Geometry: see drawing. Coordinates: mm, zero at the bounding-box minimum. A direction names the side the tool comes from. Coordinates: 2 decimals unless noted, no trailing zeros. Write each loop counter-clockwise with the first axis right and the second up, starting at its lowest first coordinate (ties: lowest second). Pieces come first, ordered by that corner, then holes.
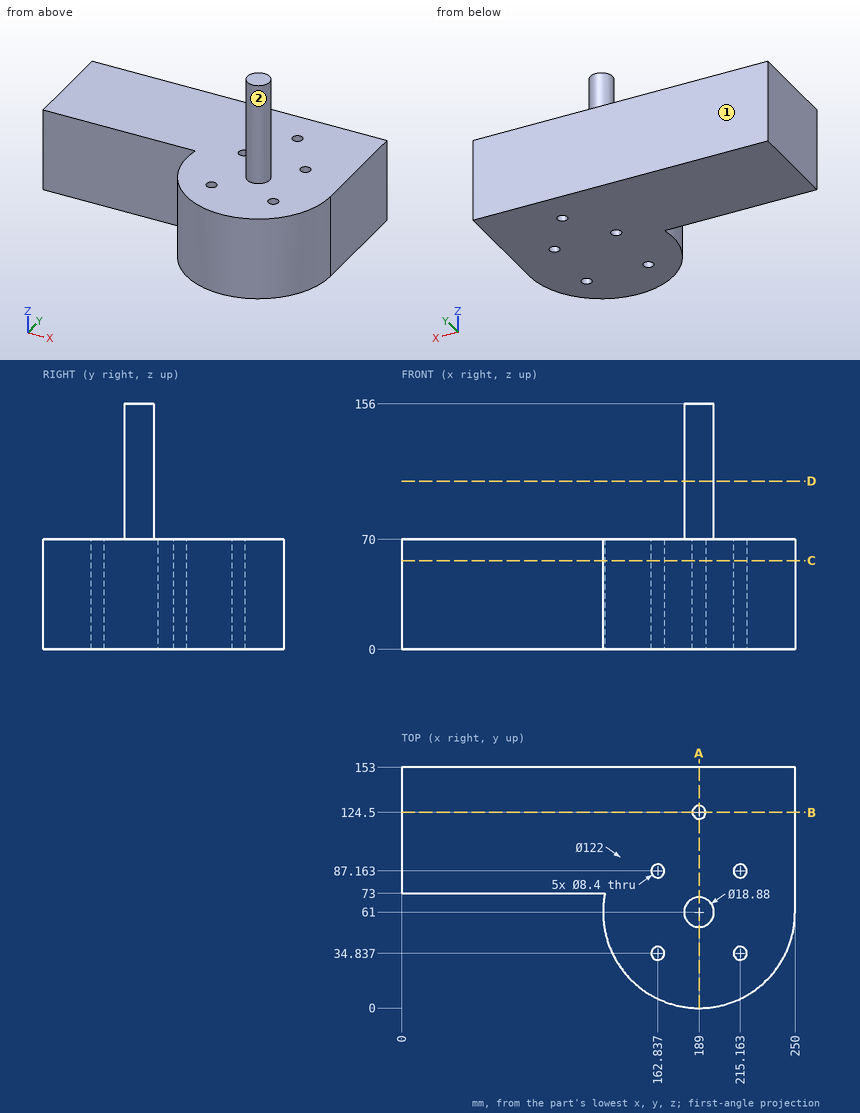
Item 1: Section A-A, the plane x = 189. Output: boundary loops of the cut face in (y, z).
Derived:
outline: (0, 0) - (120.3, 0) - (120.3, 70) - (70.44, 70) - (70.44, 156) - (51.56, 156) - (51.56, 70) - (0, 70) - close; (128.7, 0) - (153, 0) - (153, 70) - (128.7, 70) - close
Item 2: Set-up query: the marked faces 1 and 2. Return all of +Z, -Z, +X, -X, +Y, -Y with unobstructed straight access to the full face (end or side cutting, diameter ignored); none if empty.
Derived:
face 1: +Z, -Z, +X, -X, +Y
face 2: +Z
Item 3: Section D-D, the plane z = 107. Output: boundary loops of the cut face in (x, y), plus the area to 3 significant figures.
Derived:
outline: circle Ø18.88 at (189, 61)
area: 280 mm2
Item 4: Pin query (flat end, axial travel): pin 1 (13.5 mm diameter, centred on x = 215.16, y = 87.16, fed in from -Z); pin 2 (6 mm diameter, centred on x = 108, z = 36, fed in from -Y); pin 3 (1.5 mm diameter, centred on y = 58, z = 65.5, fed in from +X); pin 4 (6 mm diameter, centred on x = 33.5, y = 96.5, fed in from +Z). Return the tip coordinate at first contact, or that it passes through.
Derived:
pin 1: stops at z = 0
pin 2: stops at y = 73
pin 3: stops at x = 249.96
pin 4: stops at z = 70
Item 5: Section C-C, the plane z = 56.5. Output: boundary loops of the cut face in (x, y), plus the area to 3 significant figures.
Derived:
outline: (0, 73) - (129.19, 73) arc R61 ccw (long way) to (250, 61) - (250, 153) - (0, 153) - close; hole circle Ø8.4 at (162.84, 34.84); hole circle Ø8.4 at (162.84, 87.16); hole circle Ø8.4 at (189, 124.5); hole circle Ø8.4 at (215.16, 34.84); hole circle Ø8.4 at (215.16, 87.16)
area: 27,000 mm2
Item 6: Section B-B, the plane y = 124.5. Output: boundary loops of the cut face in (x, z), plus the area to 3 significant figures.
Derived:
outline: (0, 0) - (184.8, 0) - (184.8, 70) - (0, 70) - close; (193.2, 0) - (250, 0) - (250, 70) - (193.2, 70) - close
area: 16,900 mm2
Item 7: Material intervals for probe 1 along X at (y, z) = (87, 32); probe 2 along Y at (x, z) = (117, 41); probe 3 along Z at (x, y) = (47, 75), sorted ascending.
Derived:
probe 1: x = 0 to 158.64, 167.03 to 210.97, 219.36 to 250
probe 2: y = 73 to 153
probe 3: z = 0 to 70
